Here's the drawing with two shaded views (mm, measured from the low corner). I have some questions. Round coordinates to 2 decimals unless told otherwise and drop trailing zeros. Loops run counter-clockwise (first coordinate to the right, second up) from the corner with the lowest first, then second, coordinate; pieces in that order, holes last.
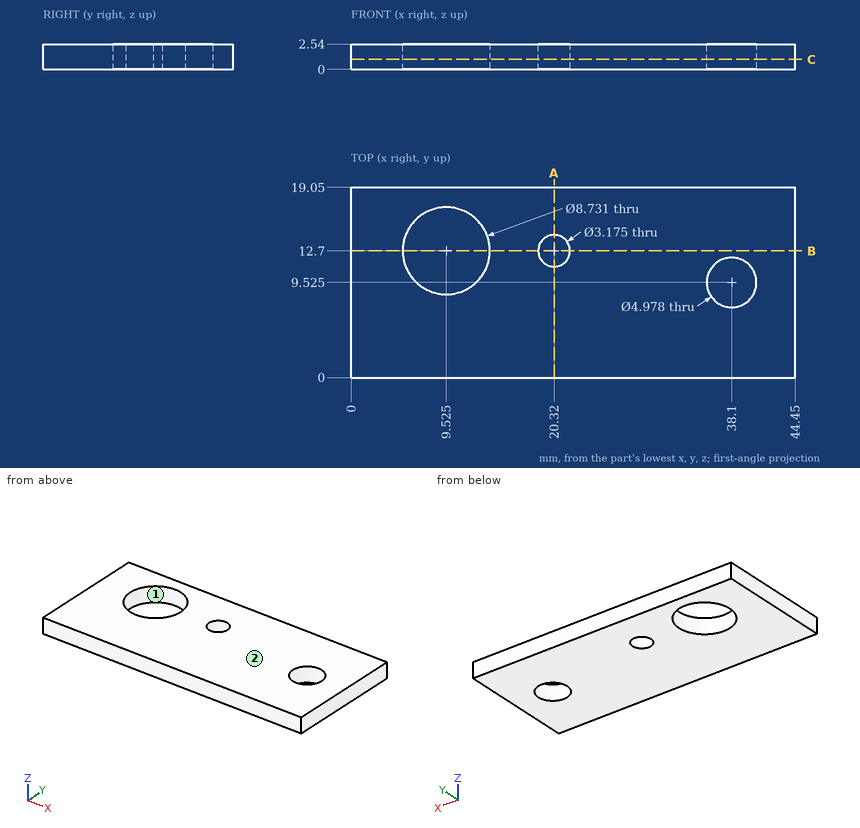
Item 1: If we section it at B-B, the plane y = 12.7: Please give me the cut outline in (x, z).
Results list:
outline: (0, 0) - (5.16, 0) - (5.16, 2.54) - (0, 2.54) - close; (13.89, 0) - (18.73, 0) - (18.73, 2.54) - (13.89, 2.54) - close; (21.91, 0) - (44.45, 0) - (44.45, 2.54) - (21.91, 2.54) - close
Item 2: If I drill on line 1 along Y through (x, z) = (20.32, 1.25); line 2 along Y through (x, z) = (38.5, 0.85); line 3 along X through (y, z) = (15.25, 2.3), over which ranges is the centre line in solid material (lowest first)?
Results list:
line 1: y = 0 to 11.11, 14.29 to 19.05
line 2: y = 0 to 7.07, 11.98 to 19.05
line 3: x = 0 to 5.98, 13.07 to 44.45
Item 3: If we section it at A-A, the plane x = 20.32: Please give me the cut outline in (y, z).
Results list:
outline: (0, 0) - (11.11, 0) - (11.11, 2.54) - (0, 2.54) - close; (14.29, 0) - (19.05, 0) - (19.05, 2.54) - (14.29, 2.54) - close
Item 4: If we section it at C-C, the plane z = 1: Count the separate pieces of the cut face and the enclosed holes in it.
Results list:
separate pieces: 1
enclosed holes: 3
Item 5: We'd pull the mould along X, two halves only. Please class the marked faces 1 and 2: released by +X, released by -X, zero draft, split by the parting line, or undercut.
Results list:
face 1: undercut
face 2: zero draft
